Design review of the part built by this model. Coordinates are the model's own, in mm. Face numbers are marked on the shaded views. A direction names the side the tool comes from. Round coordinates to 2 decimals unless told otherwise and drop trailing zeros. Write each loop counter-clockwise with the first axis right and the second up, starting at its lowest first coordinate (ties: lowest second). Pieces come first, ordered by that corner, then holes. Notation, with made-up numbers: M 47.5,52.25 L 80.5,52.25 A19 ccw 80.5,61.25 Z; hole C -19.5,67.25 d8. An arc over 180 degrees is marked long. One line per question, with ' | ' between items. Start each with the question number.
Item 1: For L1, parallel to Y at x = -3.65, z = 1.9; L2, parallel to Y at x = -3.65, z = 6.25; L3, parallel to Z at x = -135, y = 4.5, list the stretches that pass through material, from the lowest coordinate up.
Item 2: Machinability: for the marked faces 1 and 2, which of the approach directions +Z, -Z, +X, -X, +Y, -Y give a long, thin tool a straight path to every point of the face, cutting with its end or side? Answer none if there is none.
Item 3: Insertion check: pin 1 Ø1.8 at (x, y) = (-69.5, 4) entering from -Z; pin 2 Ø2.5 at (x, y) = (-2, 4.5) entering from +Z; pin 3 Ø0.5 at (x, y) = (-0.5, 3.5) entering from +Z; pin 4 Ø10 at (x, z) = (-45.5, 5.5) entering from -Y. Each pin has a flat end and moves straight along its axis. Give the tip position at first contact, or say it passes through.
Item 4: Draft analysis for pull direction X (two halves, no side actions). For the marked faces 3, 4, 5 and 6, state which applies: released by +X, released by -X, zero draft, split by the parting line, or undercut.
Item 5: Add section B-B, the plane x = -69.2. State the section outline as (y, z) points.
Item 6: Add section A-A, the plane x = -10. State the section outline as (y, z) points.
Item 7: Add section C-C, the plane x = -84.5. State the section outline as (y, z) points, and give its area (3 significant figures).
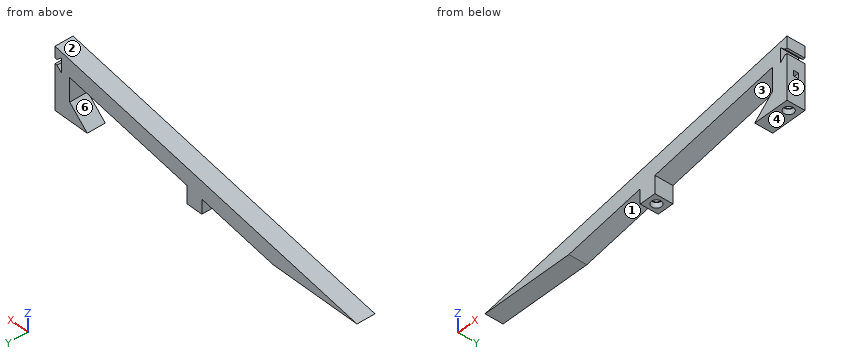
```python
from build123d import *

# Parameters (mm, degrees)
P_IDAT_VYSUNUT_M1_DEPTH  = 8
ODEBRAT_VYSUNUT_M1_DEPTH = 153.557332159
SKICA5_W                 = 16
SKICA5_H                 = 8
P_IDAT_VYSUNUT_M2_DEPTH  = 8
ODEBRAT_VYSUNUT_M4_DEPTH = 153.557332159
SKICA4_W                 = 2.4
SKICA4_H                 = 2.4
ODEBRAT_VYSUNUT_M2_DEPTH = 4.4
SKICA9_R                 = 2.2
ODEBRAT_VYSUNUT_M5_DEPTH = 2.4
SKICA10_R                = 1.85
ODEBRAT_VYSUNUT_M6_DEPTH = 7


with BuildPart() as part:
    # Skica2 → Přidat vysunutím1 (new body)
    with BuildSketch(Plane(origin=(0, 0, 0), x_dir=(1, 0, 0), z_dir=(0, 1, 0))):
        Polygon((0, 0), (0, -27.47211487), (-149.85, 0.000769495), (-108.259653873, 0.000769495), (-72.85, -6.491091207), (-72.85, 0), (-65.55, 0), (-65.55, -7.829443265), (-7.3, -18.508759343), (-7.3, 0), align=None)
    extrude(amount=P_IDAT_VYSUNUT_M1_DEPTH)

    # Skica3 → Odebrat vysunutím1 (cut, through all)
    with BuildSketch(Plane(origin=(0, 8, 0), x_dir=(1, 0, 0), z_dir=(0, 1, 0))):
        Polygon((0, -20), (-1, -20), (-3.2, -18), (-3.2, -24.4), (-1, -22.4), (0, -22.4), align=None)
    extrude(amount=-ODEBRAT_VYSUNUT_M1_DEPTH, mode=Mode.SUBTRACT)

    # Skica5 → Přidat vysunutím2 (add)
    with BuildSketch(Plane(origin=(0, 8, 0), x_dir=(1, 0, 0), z_dir=(0, 1, 0))):
        with Locations((-8, -4)):
            Rectangle(SKICA5_W, SKICA5_H)
    extrude(amount=-P_IDAT_VYSUNUT_M2_DEPTH)

    # Skica7 → Odebrat vysunutím4 (cut, through all)
    with BuildSketch(Plane.XZ):
        Polygon((-7.3, 8), (-16, 8), (-16, 0), align=None)
    extrude(amount=-ODEBRAT_VYSUNUT_M4_DEPTH, mode=Mode.SUBTRACT)

    # Skica4 → Odebrat vysunutím2 (cut)
    with BuildSketch(Plane(origin=(0, 0, 0), x_dir=(0, 0, -1), z_dir=(1, 0, 0))):
        with Locations((-13.2, 4)):
            Rectangle(SKICA4_W, SKICA4_H)
    extrude(amount=-ODEBRAT_VYSUNUT_M2_DEPTH, mode=Mode.SUBTRACT)

    # Skica9 → Odebrat vysunutím5 (cut)
    with BuildSketch(Plane(origin=(0, 0, 0), x_dir=(-1, 0, 0), z_dir=(0, 0, -1))):
        with Locations((3.65, 4)):
            Circle(SKICA9_R)
        with Locations((69.2, 4)):
            Circle(SKICA9_R)
    extrude(amount=-ODEBRAT_VYSUNUT_M5_DEPTH, mode=Mode.SUBTRACT)

    # Skica10 → Odebrat vysunutím6 (cut)
    with BuildSketch(Plane(origin=(0, 0, 2.4), x_dir=(-1, 0, 0), z_dir=(0, 0, -1))):
        with Locations((3.65, 4)):
            Circle(SKICA10_R)
        with Locations((69.2, 4)):
            Circle(SKICA10_R)
    extrude(amount=-ODEBRAT_VYSUNUT_M6_DEPTH, mode=Mode.SUBTRACT)


solid = part.part
```
Computed values:
1) L1: y = 0 to 1.8, 6.2 to 8 | L2: y = 0 to 2.15, 5.85 to 8 | L3: z = 0 to 2.72
2) face 1: -Z, +Y, -Y | face 2: +Z, -X, +Y, -Y
3) pin 1: stops at z = 9.4 | pin 2: stops at z = 27.33 | pin 3: stops at z = 27.43 | pin 4: passes through
4) face 3: undercut | face 4: zero draft | face 5: released by +X | face 6: undercut
5) outline: M 0,0 L 1.8,0 L 1.8,2.4 L 2.15,2.4 L 2.15,9.4 L 5.85,9.4 L 5.85,2.4 L 6.2,2.4 L 6.2,0 L 8,0 L 8,14.79 L 0,14.79 Z
6) outline: M 0,0 L 8,0 L 8,5.52 L 0,5.52 Z; M 0,18.01 L 8,18.01 L 8,25.64 L 0,25.64 Z
7) outline: M 0,4.36 L 8,4.36 L 8,11.98 L 0,11.98 Z | area: 61.0 mm^2
